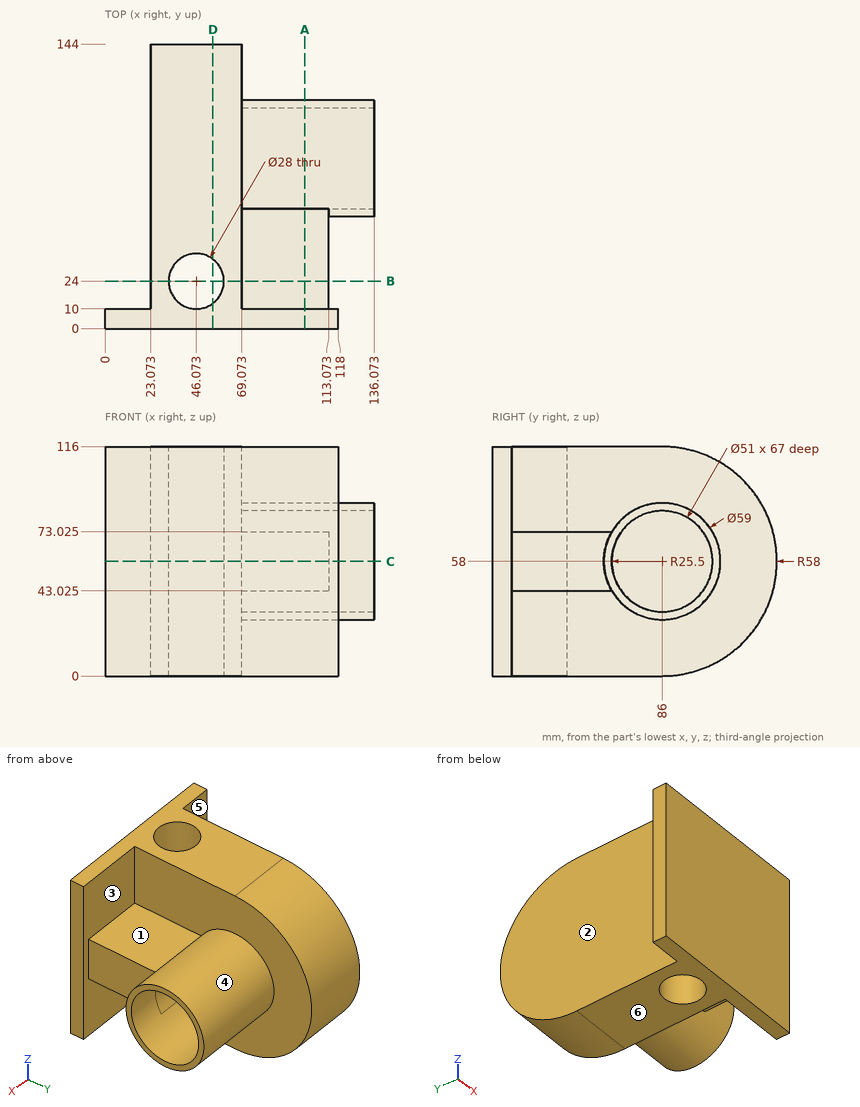
Study the drawing (mm; zero at the part's minimum x, y, z) and answer. A direction names the side the tool comes from. Give positions to 0.01 mm unless a question says otherwise; leave off trailing zeros. Loops run counter-clockwise (first coordinate to the right, second up) from the corner with the lowest first, then second, coordinate; pieces in that order, holes last. Notation, with made-up numbers: M 64,-27 L 84,-27 A7 ccw 84,-23 Z; hole C -29,-7.75 d4. An arc over 180 degrees is marked long. One line per item, written item: value.
1. For the marked faces 1, 2 and 3, determine the directions among +Z, -Z, +X, -X, +Y, -Y from which every point of the face is accessible in a straight line to the end or side of a thin tool.
Found:
face 1: +Z, +X
face 2: +Z, -Z, -X, +Y
face 3: +X
2. Section C-C on z = 58 is taken. Determine the outline of the cut face in (x, y), plus the area to 3 significant figures.
Found:
outline: M 0,0 L 118,0 L 118,10 L 113.07,10 L 113.07,56.5 L 136.07,56.5 L 136.07,60.5 L 69.07,60.5 L 69.07,111.5 L 136.07,111.5 L 136.07,115.5 L 69.07,115.5 L 69.07,144 L 23.07,144 L 23.07,10 L 0,10 Z; hole C 46.07,24 d28
area: 9,310 mm^2
3. For a pull along Y with two mould halves and no side action, classify the marked faces 4, 5 and 6 as pulls with the +Y half, pulls with the -Y half, needs draft (parallel to the pull), parting line crosses it, or undercut.
Found:
face 4: undercut
face 5: pulls with the +Y half
face 6: needs draft
4. Section B-B on y = 24 is taken. Determine the outline of the cut face in (x, z) (1 decimal).
Found:
outline: M 23.1,0 L 32.1,0 L 32.1,116 L 23.1,116 Z; M 60.1,0 L 69.1,0 L 69.1,43 L 113.1,43 L 113.1,73 L 69.1,73 L 69.1,116 L 60.1,116 Z
5. Section D-D on x = 54.5 is taken. Determine the outline of the cut face in (y, z).
Found:
outline: M 0,0 L 12.82,0 L 12.82,116 L 0,116 Z; M 35.18,0 L 86,0 A58 ccw 86,116 L 35.18,116 Z
6. Find the intervals of material crossed by probe 1 along Y at (x, z) = (122, 58); probe 2 along Z at (x, y) = (115.5, 86); probe 3 along Z at (x, y) = (95.5, 25) (1 decimal), in increasing order.
Found:
probe 1: 56.5 to 60.5, 111.5 to 115.5
probe 2: 28.5 to 32.5, 83.5 to 87.5
probe 3: 43 to 73
7. Section A-A on x = 101 is taken. Determine the outline of the cut face in (y, z) (1 decimal).
Found:
outline: M 0,0 L 10,0 L 10,43 L 60.6,43 A29.5 ccw long 60.6,73 L 10,73 L 10,116 L 0,116 Z; hole C 86,58 d51
8. Each of these flat-tipped pins is pushed along its axis until it touches: P1, Ø11.5, axis at x = 14, z = 52.5, coming from the +Y side; P2, Ø3, axis at y = 47, z = 39, coming from the -X side; P3, Ø1, axis at x = 24, z = 98.5, coming from the +Y side; P4, Ø8, axis at x = 118, z = 102.5, coming from the -Y side. Where does it stop, or does it pass through?
Found:
P1: y = 10
P2: x = 23.07
P3: y = 128
P4: y = 0
